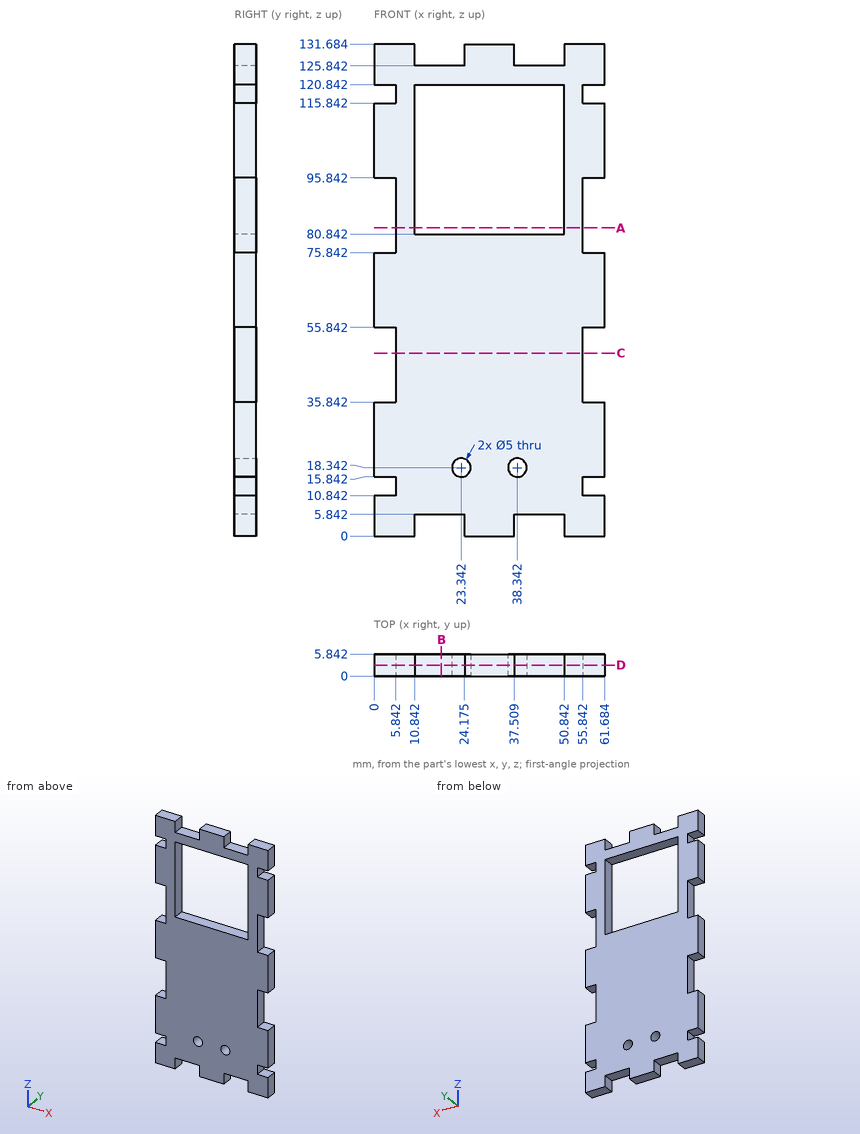
Study the drawing (mm; zero at the part's minimum x, y, z) and answer. Coordinates: 2 decimals unless noted, no trailing zeros. Write each loop counter-clockwise with the first axis right and the second up, starting at its lowest first coordinate (ties: lowest second). Pieces come first, ordered by that corner, then holes. Notation, with made-up numbers: (66.5, -31.75) -> (114.5, -31.75) arc R31 ccw to (114.5, 6.25) -> close; hole circle Ø2 at (-5.75, 63). An arc over 180 degrees is marked (long way). Write each question's results on one line, items separated by ' | '. Start each with the question number.
1) A cutting plane is placed at A-A (z = 82.5). Determine the outline of the cut face in (x, y).
2) Straight lines are drawn through the part: probe 1 along X at (y, z) = (4.4, 18) (1 decimal); probe 2 along X at (y, z) = (0.45, 99.5); probe 3 along Z at (x, y) = (57, 5.35). For each, find the intervals that lie inside material, in ascending order.
3) A cutting plane is placed at C-C (z = 49). Determine the outline of the cut face in (x, y), then the cut area to 3 significant figures.
4) Flat-ended cylindrical pins translate along their axes: pin 1 Ø1.8 at (x, y) = (15.5, 3) entering from -Z; pin 2 Ø1 at (x, y) = (21, 1) entering from +Z; pin 3 Ø1.5 at (y, z) = (2.5, 14) entering from -X. Find the tip coordinate at first contact, or state that the pin passes through.
5) A cutting plane is placed at B-B (x = 18). Determine the outline of the cut face in (y, z).
6) A cutting plane is placed at D-D (y = 2.9). Count the separate pieces of the cut face and the enclosed holes in it, then the cut area to 3 significant figures.
Values follow:
1) outline: (5.84, 0) -> (10.84, 0) -> (10.84, 5.84) -> (5.84, 5.84) -> close; (50.84, 0) -> (55.84, 0) -> (55.84, 5.84) -> (50.84, 5.84) -> close
2) probe 1: 0 to 20.9, 25.8 to 35.9, 40.8 to 61.7 | probe 2: 0 to 10.84, 50.84 to 61.68 | probe 3: 0 to 10.84, 15.84 to 35.84, 55.84 to 75.84, 95.84 to 115.84, 120.84 to 131.68
3) outline: (5.84, 0) -> (55.84, 0) -> (55.84, 5.84) -> (5.84, 5.84) -> close | area: 292 mm²
4) pin 1: z = 5.84 | pin 2: z = 125.84 | pin 3: x = 5.84
5) outline: (0, 5.84) -> (5.84, 5.84) -> (5.84, 80.84) -> (0, 80.84) -> close; (0, 120.84) -> (5.84, 120.84) -> (5.84, 125.84) -> (0, 125.84) -> close
6) separate pieces: 1 | enclosed holes: 3 | area: 5,590 mm²
